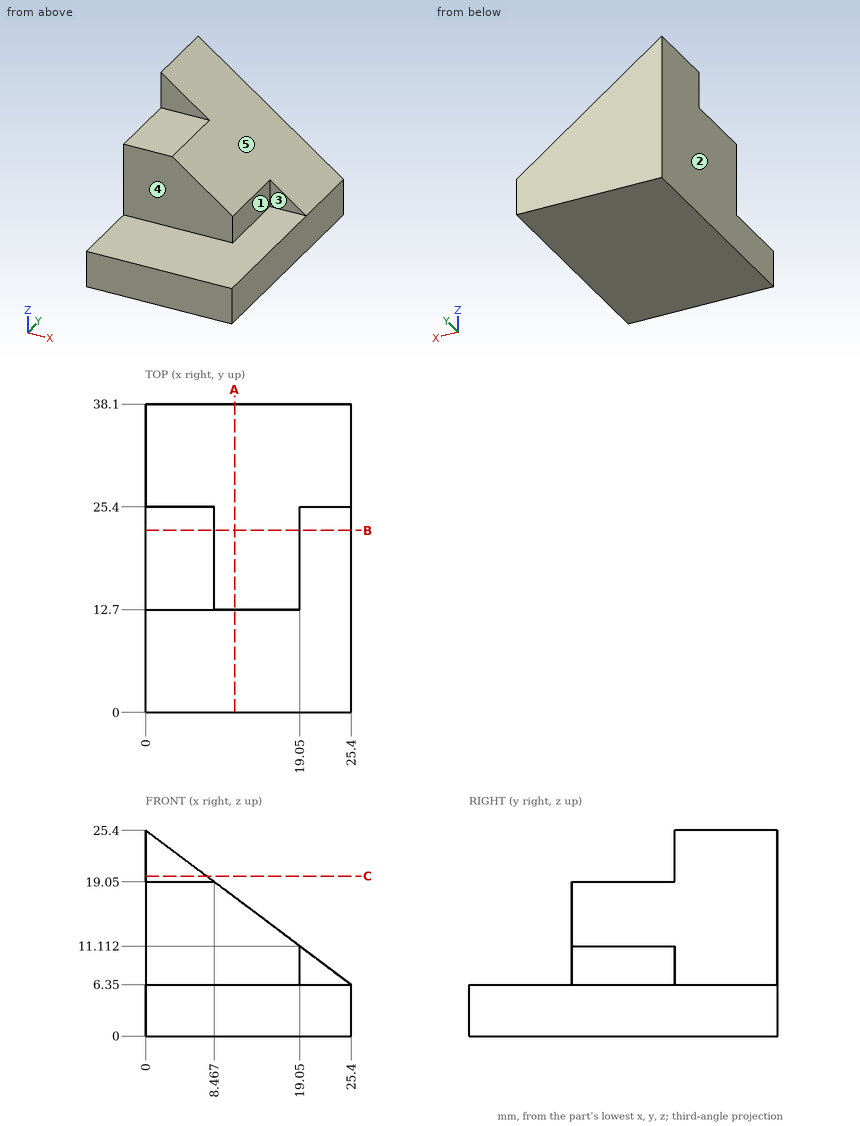
Check sheet for the drawn part. Datum: minimum x, y, z corner. Units: mm. A direction names the side the tool comes from. Give positions to 0.01 mm unless a question says otherwise; leave off trailing zeros. Loops run counter-clockwise (first coordinate to the right, second up) from the corner with the lowest first, then second, coordinate; pieces in that order, holes last. Notation, with made-up numbers: M 60.25,-28.5 L 106.25,-28.5 A23 ccw 106.25,7.5 Z; hole C 35.25,81 d10. An arc over 180 degrees is marked long. Return JSON: item names as keys, results as strings.
1) Section check C-C, the plane z = 19.75. Enter the section's corners in (x, y).
Findings:
{"outline": "M 0,25.4 L 7.53,25.4 L 7.53,38.1 L 0,38.1 Z"}
2) Tool access check on the marked faces 4 and 5. Record the directions out of +Z, -Z, +X, -X, +Y, -Y that give a thin tool (end or side, any length) a straight path to the whole face; none if there is none.
Findings:
{"face 4": "+Z, +X, -X, -Y", "face 5": "+Z, +X, +Y, -Y"}
3) Material ranges on L1, parallel to Z at x = 2.5, y = 4; L2, parallel to Y at x = 21.25, z = 7.75; L3, parallel to Y at x = 6.5, z = 13.75, recorded low to high. Write a range as [from, to].
Findings:
{"L1": "z = [0, 6.35]", "L2": "y = [25.4, 38.1]", "L3": "y = [12.7, 38.1]"}
4) Mould release check, pull along X, two halves, no side actions. Record for the marked faces 1, 2 and 3: released by +X, released by -X, zero draft, split by the parting line, or undercut.
Findings:
{"face 1": "released by +X", "face 2": "released by -X", "face 3": "zero draft"}
5) Section check B-B, the plane y = 22.5. Enter the section's corners in (x, z).
Findings:
{"outline": "M 0,0 L 25.4,0 L 25.4,6.35 L 19.05,6.35 L 19.05,11.11 L 8.47,19.05 L 0,19.05 Z"}
6) Section check A-A, the plane x = 11. Enter the section's corners in (y, z).
Findings:
{"outline": "M 0,0 L 38.1,0 L 38.1,17.15 L 12.7,17.15 L 12.7,6.35 L 0,6.35 Z"}
7) Gauge pin test, flat ends, axial feed: P1, Ø10, axis at x = 8.5, z = 12, coming from the -Y side; P2, Ø10, axis at x = 9, y = 15, coming from the +Z side; P3, Ø5, axis at x = 22.5, z = 9.5, coming from the -Y side. Record the tip position at first contact, or that the pin passes through.
Findings:
{"P1": "stops at y = 12.7", "P2": "stops at z = 19.05", "P3": "stops at y = 25.4"}
